from build123d import *

# Parameters (mm, degrees)
F0_R     = 3.175
F1_DEPTH = 44.45
F3_DEPTH = 6.35
F5_DEPTH = 6.35


with BuildPart() as f1:
    # F0 (on Right) → F1 (new body)
    with BuildSketch(Plane.YZ):
        Circle(F0_R)
    extrude(amount=F1_DEPTH)

    # F2 (on face) → F3 (cut)
    with BuildSketch(Plane.YZ.offset(44.45)):
        with BuildLine():
            ThreePointArc((2.909936, 1.27), (0, 3.175), (-2.909936, 1.27))
            Line((-2.909936, 1.27), (2.909936, 1.27))
        make_face()
    extrude(amount=-F3_DEPTH, mode=Mode.SUBTRACT)

    # F4 (on face) → F5 (cut)
    with BuildSketch(Plane(origin=(0, 0, 0), x_dir=(0, -1, 0), z_dir=(-1, 0, 0))):
        with BuildLine():
            Line((-2.909936, 1.27), (2.909936, 1.27))
            ThreePointArc((2.909936, 1.27), (0, 3.175), (-2.909936, 1.27))
        make_face()
    extrude(amount=-F5_DEPTH, mode=Mode.SUBTRACT)


solid = f1.part
Can you work these out from the model? Positions are in its coordinate system, mm. A direction names the side the tool comes from. Round coordinates to 2 decimals unless told otherwise and drop trailing zeros. Loops run counter-clockwise (first coordinate to the right, second up) from the corner with the lowest first, then second, coordinate; pieces in that order, holes last. Notation, with made-up numbers: (-39.5, 9.5) - (17.5, 9.5) arc R6 ccw to (17.5, 20.5) - close; hole circle Ø3 at (-21, -8.75). An arc over 180 degrees is marked (long way). Use CSV: the item, a comma, the result in double quotes. Start each with the question number.
1) If we section it at D-D on z = -1: Write out the boundary of the cut face in (x, y).
2) Please list where these lines run through material, in increasing order: probe 1 along Y at (x, z) = (24, -1.25); probe 2 along X at (y, z) = (-2, 1.5); probe 3 along Y at (x, z) = (21.5, 2). Write a range as [from, to].
3) If we section it at C-C on y = 2.25: Write out the boundary of the cut face in (x, z), plus the area to 3 significant figures.
4) If we section it at A-A on y = 0: Write out the boundary of the cut face in (x, z) (3 decimals), plus the area to 3 significant figures.
5) For pin 1 Ø1 at (x, z) = (23.5, -1) entering from -Y; pin 2 Ø1.5 at (x, y) = (11, -2) entering from -Z; pin 3 Ø1.7 at (x, y) = (4, -0.5) entering from +Z, each with a flat end and sliding along its axis, tell me the tip position at first contact or that it passes through.
6) For faces 1 (the flat face through (3, 0, 1.27)), 2 (the flat face through (38.1, 0, 2)), 3 (the cylindrical face through (21.91, -0.69, -3.1)), which set-ups out of +Z, -Z, +X, -X, +Y, -Y let a thin tool reach every point of the face, with its end or its side?
7) If we section it at B-B on x = 33.5: Write out the boundary of the cut face in (y, z) (3 decimals).
Geometry results:
1,outline,"(0, -3.01) - (44.45, -3.01) - (44.45, 3.01) - (0, 3.01) - close"
2,probe 1,"y = [-2.92, 2.92]"
2,probe 2,"x = [6.35, 38.1]"
2,probe 3,"y = [-2.47, 2.47]"
3,outline,"(0, -2.24) - (44.45, -2.24) - (44.45, 1.27) - (38.1, 1.27) - (38.1, 2.24) - (6.35, 2.24) - (6.35, 1.27) - (0, 1.27) - close"
3,area,"187 mm2"
4,outline,"(0, -3.175) - (44.45, -3.175) - (44.45, 1.27) - (38.1, 1.27) - (38.1, 3.175) - (6.35, 3.175) - (6.35, 1.27) - (0, 1.27) - close"
4,area,"258 mm2"
5,pin 1,"stops at y = -3.14"
5,pin 2,"stops at z = -2.92"
5,pin 3,"stops at z = 1.27"
6,face 1,"+Z, -X, +Y, -Y"
6,face 2,"+Z, +X, +Y, -Y"
6,face 3,"+X, -X"
7,outline,"circle Ø6.35 at (0, 0)"
